from build123d import *

# Parameters (mm, degrees)
SCHIZZO1_W                    = 50
SCHIZZO1_H                    = 200
ESTRUSIONE_ESTRUSIONE1_DEPTH  = 16
RACCORDO1_R                   = 5
SVUOTA1_T                     = -2
TAGLIO_ESTRUSIONE1_DEPTH      = 203.190504228
TAGLIO_ESTRUSIONE1_DEPTH_BACK = 203.190504228
SCHIZZO8_R                    = 3
TAGLIO_ESTRUSIONE2_DEPTH      = 105.312031904
SCHIZZO5_W                    = 11
SCHIZZO5_H                    = 140
TAGLIO_ESTRUSIONE3_DEPTH      = 7
SMUSSO1_SIZE                  = 2


with BuildPart() as part:
    # Schizzo1 → Estrusione-Estrusione1 (new body)
    with BuildSketch(Plane.XY):
        Rectangle(SCHIZZO1_W, SCHIZZO1_H)
    extrude(amount=ESTRUSIONE_ESTRUSIONE1_DEPTH)

    # Raccordo1
    raccordo1_edges = [part.edges().sort_by_distance(p)[0] for p in [
        (25, -100, 8),
        (-25, -100, 8),
        (-25, 100, 8),
        (25, 100, 8),
    ]]
    fillet(raccordo1_edges, radius=RACCORDO1_R)

    # Svuota1
    svuota1_openings = [part.faces().sort_by_distance(p)[0] for p in [
        (0, 0, 0),
    ]]
    offset(amount=SVUOTA1_T, openings=svuota1_openings, kind=Kind.INTERSECTION)

    # Schizzo4 → Taglio-Estrusione1 (cut, two sides: drawn at the far end of the back side and taken through both)
    with BuildSketch(Plane(origin=(0, 100, 0), x_dir=(1, 0, 0), z_dir=(0, 1, 0)).offset(-TAGLIO_ESTRUSIONE1_DEPTH_BACK)):
        Polygon((-13, 92.462112512), (-13, 0), (-13, -11), (13, -11), (13, 0), (13, 92.462112512), (13, 277.386337537), (-13, 277.386337537), align=None)
    extrude(amount=TAGLIO_ESTRUSIONE1_DEPTH + TAGLIO_ESTRUSIONE1_DEPTH_BACK, mode=Mode.SUBTRACT)

    # Schizzo8 → Taglio-Estrusione2 (cut, through all)
    with BuildSketch(Plane.XY.offset(16)):
        with Locations((-18, 93)):
            Circle(SCHIZZO8_R)
        with Locations((18, 93)):
            Circle(SCHIZZO8_R)
    taglio_estrusione2 = extrude(amount=-TAGLIO_ESTRUSIONE2_DEPTH, mode=Mode.SUBTRACT)

    # Specchia1: Taglio-Estrusione2 across plane
    add(taglio_estrusione2.mirror(Plane.ZX), mode=Mode.SUBTRACT)

    # Schizzo5 → Taglio-Estrusione3 (cut)
    with BuildSketch(Plane(origin=(25, 0, 0), x_dir=(0, 0, -1), z_dir=(1, 0, 0))):
        with Locations((-5.5, -25)):
            Rectangle(SCHIZZO5_W, SCHIZZO5_H)
    extrude(amount=-TAGLIO_ESTRUSIONE3_DEPTH, mode=Mode.SUBTRACT)

    # Smusso1
    smusso1_edges = [part.edges().sort_by_distance(p)[0] for p in [
        (15, -93, 16),
        (-21, 93, 16),
        (15, 93, 16),
        (-21, -93, 16),
    ]]
    chamfer(smusso1_edges, length=SMUSSO1_SIZE - 0.0001)  # a hair under: the kernel refuses the full size


solid = part.part
Could you check a few things on this model? Use its own coordinates, in mm. A direction names the side the tool comes from. Give positions to 0.01 mm unless a question says otherwise; leave off trailing zeros. Order: outer loops, then holes, each group sorted by start corner. A loop starts at its lowest first (then second) coordinate and runs counter-clockwise, first axis right, second up.
Item 1: I'm going to push flat-ended pins straight in: pin 1 (7 mm diameter, centred on x = -18, y = -93, fed in from +Z); pin 2 (0.6 mm diameter, centred on x = 23.5, z = 7.5, fed in from -Y); pin 3 (7 mm diameter, centred on x = -18, y = 93, fed in from -Z). Where does each tip first touch, or does it pass through?
Item 2: If we section it at D-D, the plane y = 55: Write out the boundary of the cut face in (x, z), plus the area to 3 significant figures.
Item 3: For faces 4 (the face through (24, 98, 8)), 5 (the face through (0, 98, 12)), which set-ups out of +Z, -Z, +X, -X, +Y, -Y let a thin tool reach every point of the face, with its end or its side?
Item 4: If we section it at A-A, the plane y = -93: Count the separate pieces of the cut face and the enclosed holes in it, plus the area to 3 significant figures.
Item 5: I need wall thicknesses on line 1 (X direction, y = 73, z = 1.25); line 2 (Y direction, x = -19.5, z = 3.25); line 3 (X direction, y = -93, z = 14.05). Which ranges of each line are inside material? Lowest first, please.
Item 6: If we section it at C-C, the plane z = 9.25: Write out the boundary of the cut face in (x, y), plus the area to 3 significant figures.
Item 7: If we mould it in two halves opening along X, with no side actions, what happens to faces 1 (the face through (-0.3, -100, 11.4)), 2 (the face through (-25, -1, 8)), 3 (the face through (0, 1, 14))? For each: pulls with the +X half, pulls with the -X half, needs draft (parallel to the pull), parting line crosses it, or undercut.
Values:
1. pin 1: stops at z = 14.5
1. pin 2: stops at y = -98.84
1. pin 3: stops at z = 14
2. outline: (-25, 0) - (-23, 0) - (-23, 14) - (23, 14) - (23, 0) - (25, 0) - (25, 16) - (-25, 16) - close
2. area: 156 mm2
3. face 4: +Z, -Z, +X, +Y
3. face 5: -Z
4. separate pieces: 3
4. enclosed holes: 0
4. area: 102 mm2
5. line 1: x = -25 to -23, 23 to 25
5. line 2: y = -100 to -98, 98 to 100
5. line 3: x = -25 to -21.05, -14.95 to 14.95, 21.05 to 25
6. outline: (-25, -95) arc R5 ccw to (-20, -100) - (-13, -100) - (-13, -98) - (-20, -98) arc R3 cw to (-23, -95) - (-23, 95) arc R3 cw to (-20, 98) - (-13, 98) - (-13, 100) - (-20, 100) arc R5 ccw to (-25, 95) - close; (13, -100) - (20, -100) arc R5 ccw to (25, -95) - (23, -95) arc R3 cw to (20, -98) - (13, -98) - close; (13, 98) - (20, 98) arc R3 cw to (23, 95) - (23, 45) - (25, 45) - (25, 95) arc R5 ccw to (20, 100) - (13, 100) - close
6. area: 586 mm2
7. face 1: needs draft
7. face 2: pulls with the -X half
7. face 3: undercut
